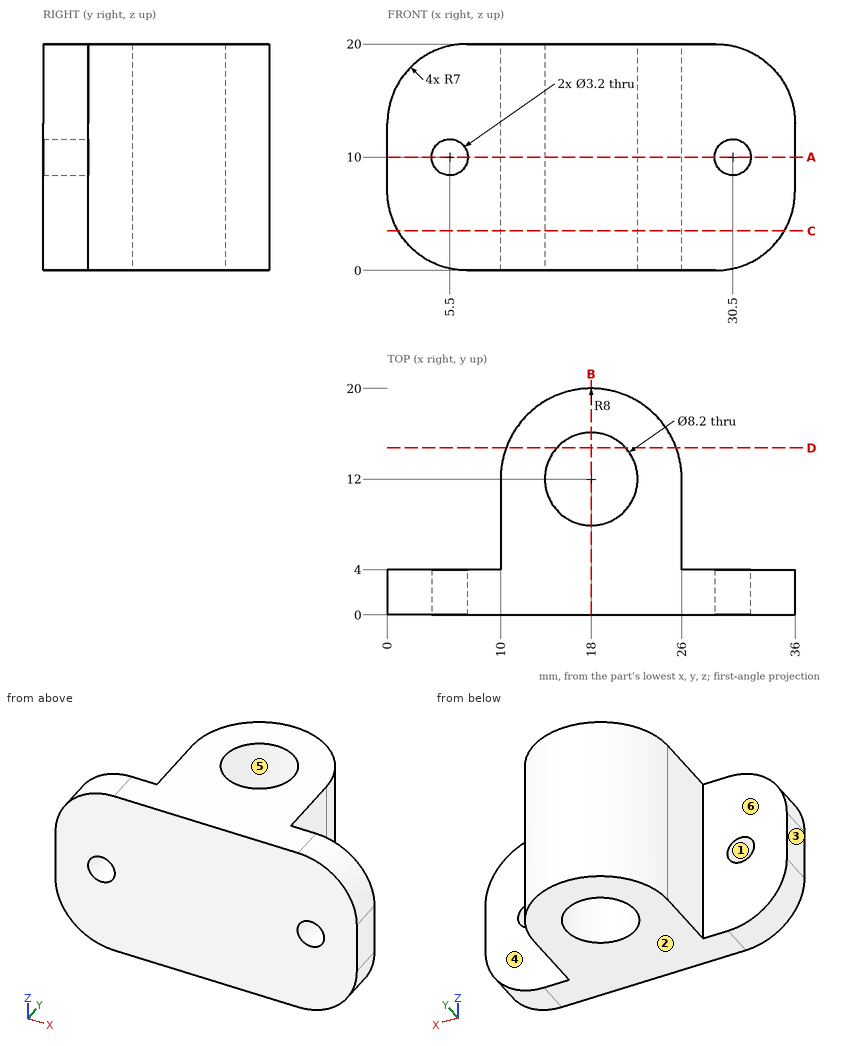
Design review of the part shown in the three views and the two pictorial views. Dimensions are in mm from the part's minimum x, y and z. A direction names the side the tool comes from. Give positions to 0.01 mm unless a question says otherwise; leave off trailing zeros. Loops run counter-clockwise (first coordinate to the right, second up) from the corner with the lowest first, then second, coordinate; pieces in that order, holes last. Notation, with made-up numbers: (-24.5, -20) - (28.5, -20) arc R25 cw to (28.5, 16) - close; hole circle Ø1 at (4.5, 22). An arc over 180 degrees is marked (long way). Write item = value, one per line.
1) Take a section at D-D on y = 14.75. State the section outline as (x, z) points, and give its area (3 significant figures).
Result sheet:
outline = (10.49, 0) - (14.96, 0) - (14.96, 20) - (10.49, 20) - close; (21.04, 0) - (25.51, 0) - (25.51, 20) - (21.04, 20) - close
area = 179 mm2
2) Take a section at B-B on x = 18. State the section outline as (y, z) points, and give its area (3 significant figures).
Result sheet:
outline = (0, 0) - (7.9, 0) - (7.9, 20) - (0, 20) - close; (16.1, 0) - (20, 0) - (20, 20) - (16.1, 20) - close
area = 236 mm2
3) Take a section at A-A on z = 10. State the section outline as (x, y) points, and give its area (3 significant figures).
Result sheet:
outline = (0, 0) - (3.9, 0) - (3.9, 4) - (0, 4) - close; (7.1, 0) - (28.9, 0) - (28.9, 4) - (26, 4) - (26, 12) arc R8 ccw to (10, 12) - (10, 4) - (7.1, 4) - close; (32.1, 0) - (36, 0) - (36, 4) - (32.1, 4) - close; hole circle Ø8.2 at (18, 12)
area = 294 mm2
4) To check wall thickness, follow line 1 (Y direction, x = 18, z = 9); line 2 (Y direction, x = 30, z = 16.25); line 3 (X direction, y = 5.25, z = 12.25). State the ranges of each line that lie inside material, in increasing order.
Result sheet:
line_1 = 0 to 7.9, 16.1 to 20
line_2 = 0 to 4
line_3 = 10 to 26
5) Tool access review of the marked faces 4, 5 and 6: name each direction out of +Z, -Z, +X, -X, +Y, -Y from which nothing blocks a thin tool from reaching the whole face with its end or side.
Result sheet:
face_4 = +Z, -Z, +X, +Y
face_5 = +Z, -Z
face_6 = +Z, -Z, -X, +Y
6) Draft analysis for pull direction Z (two halves, no side actions). For the marked faces 1, 2 and 3, state which applies: +Z half, -Z half, draft (parallel to the pull), parting line (faces both ways), or undercut.
Result sheet:
face_1 = undercut
face_2 = -Z half
face_3 = draft
7) Clearance check with flat-ended pins moving along their axes: pin 1 Ø5 at (y, z) = (11, 7.5) entering from +X; pin 2 Ø2.5 at (x, z) = (5.5, 10) entering from +Y; pin 3 Ø3 at (x, z) = (2.5, 12) entering from +Y. State where each tip first meets the part, or that it passes through.
Result sheet:
pin_1 = 26
pin_2 = through
pin_3 = 4
8) Take a section at C-C on z = 3.5. State the section outline as (x, y) points, and give its area (3 significant figures).
Result sheet:
outline = (0.94, 0) - (35.06, 0) - (35.06, 4) - (26, 4) - (26, 12) arc R8 ccw to (10, 12) - (10, 4) - (0.94, 4) - close; hole circle Ø8.2 at (18, 12)
area = 312 mm2
